Source: three-view drawing plus pictorial views. Frame: mm from the lowest corner of the part. A direction names the side the tool comes from. Coordinates: 2 decimals unless noted, no trailing zeros. Order: outer loops, then holes, each group sorted by start corner. A loop starts at its lowest first (then second) coordinate and runs counter-clockwise, first axis right, second up. Notation, with made-up numbers: (67.25, 53.5) - (122.25, 53.5) arc R22 ccw to (122.25, 62.5) - close; hole circle Ø4 at (56, 26). An arc over 180 degrees is marked (long way). One line per question, with ' | ' between items.
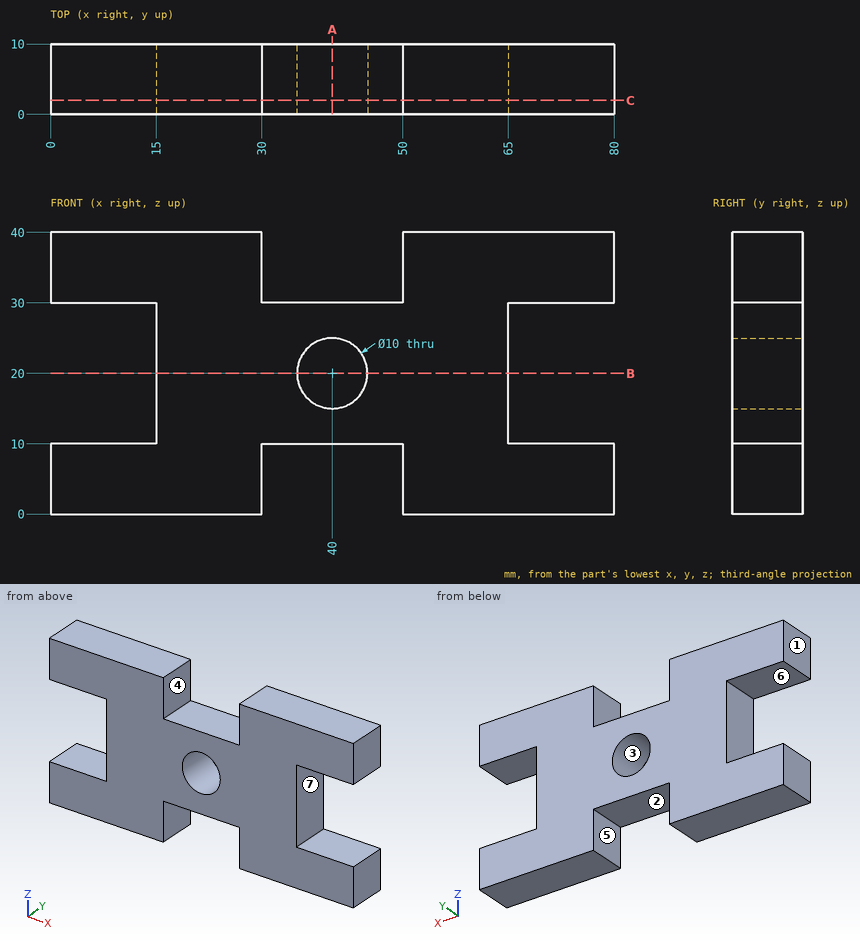
Item 1: Ray query, line 1 (Z direction, x = 75, y = 9); line 2 (Z direction, x = 40, y = 3); line 3 (X direction, y = 8, z = 9). Return the intervals inside material, ascending.
Data:
line 1: 0 to 10, 30 to 40 | line 2: 10 to 15, 25 to 30 | line 3: 0 to 30, 50 to 80
Item 2: Section B-B on z = 20. Return the cut outline in (x, y).
Data:
outline: (15, 0) - (35, 0) - (35, 10) - (15, 10) - close; (45, 0) - (65, 0) - (65, 10) - (45, 10) - close
Item 3: Section C-C on y = 2. Return the cut outline in (x, z).
Data:
outline: (0, 0) - (30, 0) - (30, 10) - (50, 10) - (50, 0) - (80, 0) - (80, 10) - (65, 10) - (65, 30) - (80, 30) - (80, 40) - (50, 40) - (50, 30) - (30, 30) - (30, 40) - (0, 40) - (0, 30) - (15, 30) - (15, 10) - (0, 10) - close; hole circle Ø10 at (40, 20)
Item 4: Draft query along Z for the marked faces 1, 2 and 3. Return one class per face: released by +Z, released by -Z, zero draft, split by the parting line, or undercut.
Data:
face 1: zero draft | face 2: released by -Z | face 3: undercut
Item 5: Access query for the marked faces 4, 5, 6 and 7. Directions: +Z, -Z, +X, -X, +Y, -Y. A direction counts if a zero-diameter tool reaches every point of the face in a straight line with its end or side. Return the directions, or none.
Data:
face 4: +Z, +Y, -Y | face 5: -Z, +Y, -Y | face 6: -X, +Y, -Y | face 7: +X, +Y, -Y
Item 6: Section A-A on x = 40. Return the cut outline in (y, z).
Data:
outline: (0, 10) - (10, 10) - (10, 15) - (0, 15) - close; (0, 25) - (10, 25) - (10, 30) - (0, 30) - close
Item 7: Contact query for flat-ended pins moving along their axis: P1, Ø5, axis at x = 37.5, y = 5.5, coming from the -Z side; P2, Ø3, axis at y = 5.5, z = 17, coming from the +X side. Output: stop coordinate, or through.
Data:
P1: z = 10 | P2: x = 65
